```python
from build123d import *

# Parameters (mm, degrees)
F0_W     = 19.05
F0_H     = 127
F1_DEPTH = 76.2
F2_W     = 76.2
F2_H     = 19.05
F3_DEPTH = 8.89
F4_R     = 5.07999


# Not quite as in the source:
# - a fillet or chamfer is up to 0.001 mm smaller than in the source, because OpenCascade refuses the exact size


with BuildPart() as f1:
    # F0 (on Front) → F1 (new body)
    with BuildSketch(Plane.XZ):
        with Locations((-61.3191734314, 10.0326964855)):
            Rectangle(F0_W, F0_H)
    extrude(amount=F1_DEPTH)

    # F2 (on face) → F3 (cut)
    with BuildSketch(Plane.YZ.offset(-51.7941734314)):
        with Locations((-38.1, 47.7159310818)):
            Rectangle(F2_W, F2_H)
    extrude(amount=-F3_DEPTH, mode=Mode.SUBTRACT)

    # F4 (radius 5.08 in the source; OpenCascade refuses exactly that, so slightly less here)
    f4_edges = [f1.edges().sort_by_distance(p)[0] for p in [
        (-70.844173, -76.2, 10.032696),
        (-51.794173, -76.2, 65.386814),
        (-61.319173, -76.2, 73.532696),
        (-60.684173, -76.2, 47.715931),
        (-60.684173, 0, 47.715931),
        (-51.794173, -76.2, -7.638186),
        (-51.794173, -38.1, -53.467304),
        (-61.319173, -76.2, -53.467304),
        (-61.319173, 0, -53.467304),
        (-51.794173, 0, -7.638186),
        (-70.844173, 0, 10.032696),
        (-51.794173, 0, 65.386814),
        (-61.319173, 0, 73.532696),
        (-51.794173, -38.1, 73.532696),
        (-70.844173, -38.1, 73.532696),
    ]]
    fillet(f4_edges, radius=F4_R)


solid = f1.part
```
Can you work these out from the model? Positions are in its coordinate system, mm. A direction names the side the tool comes from. Round coordinates to 2 decimals unless told otherwise and drop trailing zeros. Loops run counter-clockwise (first coordinate to the right, second up) from the corner with the lowest first, then second, coordinate; pieces in that order, holes last. Notation, with made-up numbers: (85, 30.5) -> (102, 30.5) arc R22 cw to (102, 68.5) -> close; hole circle Ø11 at (-3, -27.5). An arc over 180 degrees is marked (long way). Answer in a Markdown table with one row per item.
Item 1: Suppose I cut it at C-C, the plane x = -55.25. List the corners of the cut face in (y, z) for me.
Answer block:
| item | result |
|---|---|
| outline | (-75.93, -48.39) arc R4.81 ccw to (-71.12, -53.2) -> (-5.08, -53.2) arc R4.81 ccw to (-0.27, -48.39) -> (-0.27, 38.19) -> (-75.93, 38.19) -> close; (-75.93, 57.24) -> (-0.27, 57.24) -> (-0.27, 68.45) arc R4.81 ccw to (-5.08, 73.27) -> (-71.12, 73.27) arc R4.81 ccw to (-75.93, 68.45) -> close |
Item 2: Suppose I cut it at D-D, the plane x = -69. List the corners of the cut face in (y, z) for me, plus the area to 3 significant figures.
Answer block:
| item | result |
|---|---|
| outline | (-75.04, -51.62) arc R5.08 ccw to (-71.12, -53.47) -> (-5.08, -53.47) arc R5.08 ccw to (-1.16, -51.62) -> (-1.16, 68.45) arc R3.92 ccw to (-5.08, 72.37) -> (-71.12, 72.37) arc R3.92 ccw to (-75.04, 68.45) -> close |
| area | 9,280 mm² |
Item 3: If I drill on probe 1 along Z at (x, y) = (-59.5, -63); probe 2 along X at (y, z) = (-33.5, 45.5); probe 3 along Z at (x, y) = (-66, -70), over which ranges is the centre line in solid material (lowest first)?
Answer block:
| item | result |
|---|---|
| probe 1 | -53.47 to 38.19, 57.24 to 73.53 |
| probe 2 | -70.84 to -60.68 |
| probe 3 | -53.47 to 73.53 |
Item 4: Suppose I cut it at A-A, the plane z = -24.5. List the corners of the cut face in (x, y) for me, plus the area to 3 significant figures.
Answer block:
| item | result |
|---|---|
| outline | (-70.84, -71.12) arc R5.08 ccw to (-65.76, -76.2) -> (-56.87, -76.2) arc R5.08 ccw to (-51.79, -71.12) -> (-51.79, -5.08) arc R5.08 ccw to (-56.87, 0) -> (-65.76, 0) arc R5.08 ccw to (-70.84, -5.08) -> close |
| area | 1,430 mm² |
Item 5: On a 3-axis mill with a long thin cutter (end or side, diameter ignored), from which of +Z, -Z, +X, -X, +Y, -Y can I reach the whole of each face in a straight line? I mean faces 1 (the cylindrical face through (-61.257, -74.672, 72.084)), 2 (the cylindrical face through (-62.21, -74.75, 47.85)), 3 (the flat face through (-60.684, -39, 48)). Say none if no direction works.
Answer block:
| item | result |
|---|---|
| face 1 | +Z, +X, -X, -Y |
| face 2 | +X, -Y |
| face 3 | +X, +Y, -Y |
Item 6: Suppose I cut it at B-B, the plane y = -34.5. List the corners of the cut face in (x, z) for me.
Answer block:
| item | result |
|---|---|
| outline | (-70.84, -53.47) -> (-56.87, -53.47) arc R5.08 ccw to (-51.79, -48.39) -> (-51.79, 38.19) -> (-60.68, 38.19) -> (-60.68, 57.24) -> (-51.79, 57.24) -> (-51.79, 68.45) arc R5.08 ccw to (-56.87, 73.53) -> (-65.76, 73.53) arc R5.08 ccw to (-70.84, 68.45) -> close |
Item 7: We'd pull the mould along Z, two halves only. Please class faces 4 (the cylindrical face through (-63.76, -1.53, -52.02)), 5 (the flat face through (-57, -39, 38.191)), 6 (the cylindrical face through (-61.257, -1.528, 72.084)): released by +Z, released by -Z, zero draft, split by the parting line, or undercut.
Answer block:
| item | result |
|---|---|
| face 4 | released by -Z |
| face 5 | undercut |
| face 6 | released by +Z |
Item 8: Will this pin go through, and if not, where does the flat tip stop? P1, Ø2, axis at y = -56.5, z = 49.5, coming from the +X side.
Answer block:
| item | result |
|---|---|
| P1 | x = -60.68 |
